Geometry: final body of the model. Coordinates: model frame, mm. Face numbers are marked on the shaded views. A direction names the side the tool comes from. Coordinates: 2 decimals unless noted, no trailing zeros. Loops run counter-clockwise (first coordinate to the right, second up) from the corner with the lowest first, then second, coordinate; pieces in that order, holes last. Notation, with made-up numbers: (66, 46) - (110, 46) arc R27 ccw to (110, 85) - close; hole circle Ø2 at (60, 34.25). An arc over 180 degrees is marked (long way). Put each result on its own line as item: value. Start each with the question number.
1) Material intervals for line 1 along Y through (x, z) = (2.75, 1.25); line 2 along Y through (x, z) = (-0.25, -4); line 3 along Y through (x, z) = (-1.5, 5), sorted ascending. Write a range as from..to.
2) Section B-B on x = 3. Output: boundary loops of the cut face in (y, z), and give its area (3 significant figures).
3) Section D-D on z = 0.25. Output: boundary loops of the cut face in (x, y).
4) Section A-A on z = 5. Output: boundary loops of the cut face in (x, y), and give its area (3 significant figures).
5) Reachability of the marked faces 1, 2 and 3 from +Z, -Z, +X, -X, +Y, -Y: full face, straight path, thin tool, end or side. Return the list, or none.
6) Draft query along X for the marked faces 4, 5 and 6. Return one class per face: +X half, -X half, draft (parallel to the pull), parting line (faces both ways), or undercut.
7) Contact query for flat-ended pins moving along their axis: pin 1 Ø1.5 at (x, y) = (2, 3.5) entering from -Z; pin 2 Ø1.1 at (y, z) = (5, -6.5) entering from +X; pin 3 Ø3 at (y, z) = (2, 4) entering from +X; pin 4 Ø4.5 at (x, z) = (0, -1) entering from -Y. Output: stop coordinate, or through.
8) Section C-C on y = 4.75. Output: boundary loops of the cut face in (x, z), and give its area (3 significant figures).
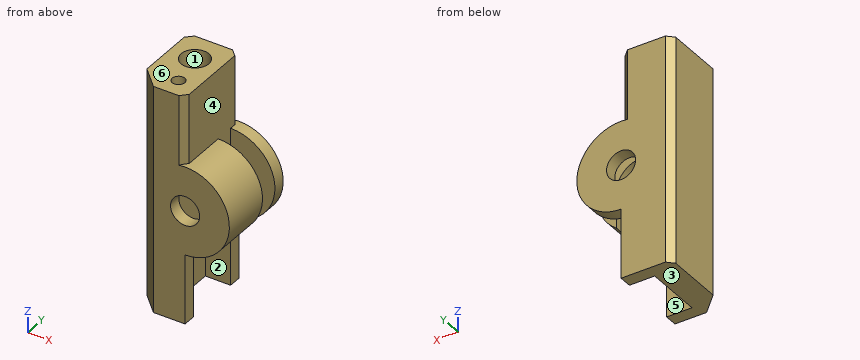
Autodesk Inventor part; units mm, degrees
ref_plane "YZ Plane" through (0, 0, 0) normal (1, 0, 0) x (0, 1, 0)
ref_plane "XZ Plane" through (0, 0, 0) normal (0, 1, 0) x (-1, 0, 0)
ref_plane "XY Plane" through (0, 0, 0) normal (0, 0, 1) x (1, 0, 0)
sketch "スケッチ1" plane through (0, 0, 0) normal (0, 1, 0) x (-1, 0, 0)
  circle A0 centre (0, 0) radius 1.15
  circle A1 centre (0, 0) radius 2
  circle A2 centre (0, 0) radius 3.5
  line L0 (0, 0) -> (0, 3.5)
  line L1 (2, 0) -> (-2, 0)
  line L2 (2, 0) -> (2, -2.8723)
  line L3 (-2, 0) -> (-2, -2.8723)
  line L4 (0, 2) -> (3.5, 2)
  line L5 (3.5, 2) -> (3.5, 6)
  line L6 (3.5, 6) -> (0, 6)
  line L7 (0, 6) -> (0, 2)
  line L8 (0, 6) -> (3.5, 6)
  line L9 (3.5, 6) -> (3.5, 0)
  line L10 (3.5, 0) -> (0, 0)
  line L11 (0, 0) -> (0, 6)
  line L12 (0, 0) -> (0, -8)
  line L13 (0, 0) -> (3.5, 0)
  line L14 (3.5, 0) -> (3.5, -8)
  line L15 (3.5, -8) -> (0, -8)
  line L16 (0, -8) -> (0, 0)
  line L17 (2, -2.8723) -> (2, -8)
  line L18 (0, -8) -> (3.5, -4.5)
  line L19 (0, -8) -> (4.9497, -8) construction
  line L20 (0, 0) -> (3.5, 0)
  line L21 (3.5, 0) -> (3.5, -9)
  line L22 (3.5, -9) -> (0, -9)
  line L23 (0, -9) -> (0, 0)
  line L24 (0, 2) -> (4, 2)
  line L25 (4, 2) -> (4, 9)
  line L26 (4, 9) -> (0, 9)
  line L27 (0, 9) -> (0, 2)
  line L28 (0, 9) -> (4, 9)
  line L29 (4, 9) -> (4, -9)
  line L30 (4, -9) -> (0, -9)
  line L31 (0, -9) -> (0, 9)
  line L32 (0, 0) -> (2, 0)
  line L33 (2, 0) -> (2, -9)
  line L34 (2, -9) -> (0, -9)
  line L35 (0, -9) -> (0, 0)
  point P0 (2, -6)
  point P1 (0, -3.5)
  dimension "d0" = 2.3
  dimension "d1" = 4
  dimension "d2" = 7
  dimension "d3" = 3.5
  dimension "d4" = 4
  dimension "d5" = 8
  dimension "d6" = 45
  dimension "d40" = 9
  dimension "d41" = 4
  dimension "d42" = 7
extrude "押し出し1" add sketch "スケッチ1" along normal blind 3 contours A1 L3 A2 L0
extrude "押し出し2" add sketch "スケッチ1" along normal blind 4.5 contours L10 A2 L2 | A1 L4 A2 L10 | L0 A2 L4 | A2 L14 L18 L17 | A2 L4 L9 | L9 L24 L29 L30 L21 L14 | L7 L6 L5 L4 A2 | L18 L14 L15 L17 | L5 L6 L27 L26 L25 L24 | L15 L21 L22 L33
extrude "押し出し3" add sketch "スケッチ1" against normal blind 1 contours L1 A1 L12 A0 | A0 L0 A1 L1 | A0 L1 A1 L0 | L12 A1 L1 A0 | L2 A2 L12 A1 | L10 A2 L2 | A1 L4 A2 L10 | A1 L3 A2 L0 | L0 A2 L4 | L12 A2 L3 A1 | L17 L18 L12 A2 | A2 L14 L18 L17 | A2 L4 L9 | L9 L24 L29 L30 L21 L14 | L7 L6 L5 L4 A2 | L18 L14 L15 L17 | L17 L15 L18 | L5 L6 L27 L26 L25 L24 | L15 L33 L22 L23 | L15 L21 L22 L33
sketch "スケッチ4" plane through (0, 4.5, 0) normal (0, 1, 0) x (1, 0, 0)
  circle A0 centre (0, 0) radius 1.15
  circle A1 centre (0, 0) radius 2
  circle A2 centre (0, 0) radius 3.5
  line L0 (-4, 9) -> (-4, -9)
  line L1 (0, 0) -> (-4, 0)
  line L2 (-4, 0) -> (-4, -9)
  line L3 (-4, -9) -> (0, -9)
  line L4 (0, -9) -> (0, 0)
  line L5 (0, 0) -> (-4, 0)
  line L6 (-4, 0) -> (-4, 9)
  line L7 (-4, 9) -> (0, 9)
  line L8 (0, 9) -> (0, 0)
  point P0 (0, -3.5)
  point P1 (0, 3.5)
  dimension "d43" = 2.3
  dimension "d44" = 4
  dimension "d45" = 7
  dimension "d46" = 4
  dimension "d47" = 9
extrude "押し出し6" add sketch "スケッチ4" along normal blind 1 contours A0 L8 A1 L4 | A0 L1 A1 L8 | L4 A1 L1 A0 | L8 A2 L4 A1 | A1 L1 A2 L8 | L4 A2 L1 A1 | A2 L1 L0 L7 L8 | L4 L3 L0 L1 A2
sketch "スケッチ5" plane through (-4, -1, 9) normal (0, 0, 1) x (1, 0, 0)
  line L0 (4, 0) -> (4, 4)
  line L1 (4, 0) -> (0, 0)
  line L2 (0, 0) -> (0, 1)
  line L3 (0, 1) -> (4, 1)
  line L4 (4, 1) -> (4, 0)
  line L5 (4, 1) -> (2.5, 1)
  line L6 (2.5, 1) -> (2.5, 1.5)
  line L7 (2.5, 1.5) -> (4, 1.5)
  line L8 (4, 1.5) -> (4, 1)
  line L9 (4, 6.5) -> (0, 6.5)
  line L10 (0, 6.5) -> (2, 6.5)
  line L11 (2, 6.5) -> (2, 4.25)
  line L12 (2, 4.25) -> (0, 4.25)
  line L13 (0, 4.25) -> (0, 6.5)
  circle A0 centre (2, 4.25) radius 1.1
  dimension "d50" = 4
  dimension "d51" = 1
  dimension "d52" = 1.5
  dimension "d53" = 0.5
  dimension "d54" = 2
  dimension "d55" = 2.25
  dimension "d56" = 2.2
extrude "押し出し7" cut sketch "スケッチ5" against normal blind 7 contours A0 L12 L11 | L11 L12 A0
hole "穴2" at (-1.5, 0.5, 9) direction (0, 0, -1) diameter 1 end through all
chamfer "面取り1" distance 0.5 angle 45 3 edges at (0, -1, 6.25) (0, 5.5, 6.25) (-4, 5.5, 0)
chamfer "面取り2" distance 1.5 angle 45 1 edges at (-4, -1, 0)
properties part number "rod6.1"
Answer block:
1. line 1: y = -1..3, 4.5..5.5
1. line 2: y = -1..0, 4.5..5.5
1. line 3: y = -1..0, 1..2.27, 4.23..5.5
2. outline: (-1, -1.8) - (3, -1.8) - (3, 1.8) - (-1, 1.8) - close; (4.5, -1.8) - (5.5, -1.8) - (5.5, 1.8) - (4.5, 1.8) - close
2. area: 18.0 mm²
3. outline: (-4, 0.5) - (-2.5, -1) - (-1.12, -1) - (-1.12, 0) - (-1.98, 0) - (-1.98, 0.38) arc R0.5 cw to (-1.98, 0.62) - (-1.98, 4.5) - (-1.12, 4.5) - (-1.12, 5.5) - (-3.5, 5.5) - (-4, 5) - close; (1.12, -1) - (3.49, -1) - (3.49, 3) - (1.98, 3) - (1.98, 0) - (1.12, 0) - close; (1.12, 4.5) - (3.49, 4.5) - (3.49, 5.5) - (1.12, 5.5) - close
4. outline: (-4, 0.5) - (-2.5, -1) - (-0.5, -1) - (0, -0.5) - (0, 5) - (-0.5, 5.5) - (-3.5, 5.5) - (-4, 5) - close; hole circle Ø2.2 at (-2, 3.25); hole circle Ø1 at (-1.5, 0.5)
4. area: 19.9 mm²
5. face 1: +Z
5. face 2: -Z, +X
5. face 3: -Z, +X, -X, +Y, -Y
6. face 4: +X half
6. face 5: undercut
6. face 6: draft
7. pin 1: stops at z = -2.87
7. pin 2: stops at x = 0
7. pin 3: stops at x = 2.45
7. pin 4: stops at y = -1
8. outline: (-4, -9) - (0, -9) - (0, -3.5) arc R3.5 ccw to (0, 3.5) - (0, 9) - (-4, 9) - close; hole circle Ø2.3 at (0, 0)
8. area: 87.1 mm²
